For this review, take the finished solid that the model builds, in its own axes (mm). Face numbers are marked on the shaded views. A direction names the side the tool comes from. Coordinates: 2 decimals unless noted, no trailing zeros. Order: outer loops, then holes, each group sorted by start corner. A loop starts at its lowest first (then second) coordinate and runs counter-clockwise, first axis right, second up. Notation, with made-up numbers: (44, 4) -> (51, 4) arc R21 ccw to (51, 11) -> close; hole circle Ø5 at (29, 39.25). An arc over 180 degrees is marked (long way). Answer as a JSON object with one key per item and string values. Group by question number.
1) Machinability: for the marked faces 1, 2 and 3, which of the approach directions +Z, -Z, +X, -X, +Y, -Y give a long, thin tool a straight path to every point of the face, cutting with its end or side? Answer none if there is none.
2) For pin 1 (3 mm diameter, centred on x = 12, z = -2, fed in from +Y); pin 2 (3 mm diameter, centred on x = 15.5, y = 1, fed in from +Z); pin 3 (4 mm diameter, centred on x = 6, y = 1.5, fed in from +Z), all flat-tipped, find the tip position at first contact; note any pin that passes through.
3) Wall thickness on L1, parallel to X at y = -2.5, z = -0.75; L2, parallel to X at y = 2, z = -2.5; L3, parallel to Z at x = 5.75, y = -2.5: over which ranges is each line inside the solid? List them lowest first.
4) Add section C-C, the plane x = 10. Write out the cut boundary in (y, z).
5) Add section D-D, the plane x = -0.75. Write out the cut boundary in (y, z).
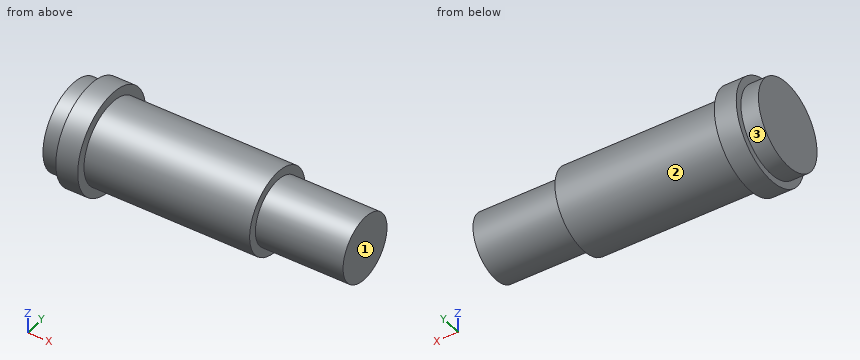
from build123d import *

# Parameters (mm, degrees)
SKETCH2_R          = 6.35
CUT_EXTRUDE1_DEPTH = 4.4925


with BuildPart() as part:
    # Sketch1 → Revolve1 (revolve)
    with BuildSketch(Plane.XY):
        Polygon((-6.35, 0), (18.35, 0), (18.35, 2.38125), (12, 2.38125), (12, 3), (0, 3), (0, 3.683), (-1.5875, 3.683), (-1.5875, 3.175), (-6.35, 3.175), align=None)
    revolve(axis=Axis((-160.130718954, 0, 0), (1, 0, 0)))

    # Sketch2 → Cut-Extrude1 (cut, through all)
    with BuildSketch(Plane(origin=(-2.8575, -8.19662542, -7.078645384), x_dir=(0, -0.923004378, -0.384789447), z_dir=(1, 0, 0))):
        with Locations((-10.289309191, -3.379645711)):
            Circle(SKETCH2_R)
    extrude(amount=-CUT_EXTRUDE1_DEPTH, mode=Mode.SUBTRACT)


solid = part.part
Output values:
{
 "1": {"face 1": "+Z, -Z, +X, +Y, -Y", "face 2": "+X", "face 3": "-X"},
 "2": {"pin 1": "stops at y = 2.96", "pin 2": "stops at z = 2.38", "pin 3": "stops at z = 3"},
 "3": {"L1": "x = -2.86 to 12", "L2": "x = -1.59 to 0", "L3": "z = -1.66 to 1.66"},
 "4": {"outline": "circle Ø6 at (0, 0)"},
 "5": {"outline": "circle Ø7.37 at (0, 0)"}
}
